```python
from build123d import *

# Parameters (mm, degrees)
SKETCH1_W           = 322.22857931
SKETCH1_H           = 163.1
BOSS_EXTRUDE1_DEPTH = 6.35
SKETCH2_R           = 10.775
CUT_EXTRUDE1_DEPTH  = 362.210727726


with BuildPart() as part:
    # Sketch1 → Boss-Extrude1 (new body)
    with BuildSketch(Plane.XY):
        with Locations((161.114289655, 81.55)):
            Rectangle(SKETCH1_W, SKETCH1_H)
    extrude(amount=BOSS_EXTRUDE1_DEPTH)

    # Sketch2 → Cut-Extrude1 (cut, through all)
    with BuildSketch(Plane.XY.offset(6.35)):
        with Locations((28.8625, 21.55)):
            Circle(SKETCH2_R)
        with Locations((40.366079306, 45.544994544)):
            Circle(SKETCH2_R)
        with Locations((51.8625, 21.55)):
            Circle(SKETCH2_R)
        with Locations((74.8625, 21.55)):
            Circle(SKETCH2_R)
        with Locations((97.8625, 21.55)):
            Circle(SKETCH2_R)
        with Locations((120.8625, 21.55)):
            Circle(SKETCH2_R)
        with Locations((143.8625, 21.55)):
            Circle(SKETCH2_R)
        with Locations((166.8625, 21.55)):
            Circle(SKETCH2_R)
        with Locations((189.8625, 21.55)):
            Circle(SKETCH2_R)
        with Locations((212.8625, 21.55)):
            Circle(SKETCH2_R)
        with Locations((235.8625, 21.55)):
            Circle(SKETCH2_R)
        with Locations((258.8625, 21.55)):
            Circle(SKETCH2_R)
        with Locations((281.8625, 21.55)):
            Circle(SKETCH2_R)
        with Locations((293.366079306, 45.544994544)):
            Circle(SKETCH2_R)
        with Locations((293.366079306, 93.544994544)):
            Circle(SKETCH2_R)
        with Locations((293.366079306, 141.544994544)):
            Circle(SKETCH2_R)
        with Locations((28.8625, 117.55)):
            Circle(SKETCH2_R)
        with Locations((28.8625, 69.55)):
            Circle(SKETCH2_R)
        with Locations((63.366079306, 45.544994544)):
            Circle(SKETCH2_R)
        with Locations((86.366079306, 45.544994544)):
            Circle(SKETCH2_R)
        with Locations((109.366079306, 45.544994544)):
            Circle(SKETCH2_R)
        with Locations((132.366079306, 45.544994544)):
            Circle(SKETCH2_R)
        with Locations((155.366079306, 45.544994544)):
            Circle(SKETCH2_R)
        with Locations((178.366079306, 45.544994544)):
            Circle(SKETCH2_R)
        with Locations((201.366079306, 45.544994544)):
            Circle(SKETCH2_R)
        with Locations((224.366079306, 45.544994544)):
            Circle(SKETCH2_R)
        with Locations((247.366079306, 45.544994544)):
            Circle(SKETCH2_R)
        with Locations((270.366079306, 45.544994544)):
            Circle(SKETCH2_R)
        with Locations((51.8625, 69.55)):
            Circle(SKETCH2_R)
        with Locations((74.8625, 69.55)):
            Circle(SKETCH2_R)
        with Locations((97.8625, 69.55)):
            Circle(SKETCH2_R)
        with Locations((120.8625, 69.55)):
            Circle(SKETCH2_R)
        with Locations((143.8625, 69.55)):
            Circle(SKETCH2_R)
        with Locations((166.8625, 69.55)):
            Circle(SKETCH2_R)
        with Locations((189.8625, 69.55)):
            Circle(SKETCH2_R)
        with Locations((212.8625, 69.55)):
            Circle(SKETCH2_R)
        with Locations((235.8625, 69.55)):
            Circle(SKETCH2_R)
        with Locations((258.8625, 69.55)):
            Circle(SKETCH2_R)
        with Locations((281.8625, 69.55)):
            Circle(SKETCH2_R)
        with Locations((51.8625, 117.55)):
            Circle(SKETCH2_R)
        with Locations((74.8625, 117.55)):
            Circle(SKETCH2_R)
        with Locations((97.8625, 117.55)):
            Circle(SKETCH2_R)
        with Locations((120.8625, 117.55)):
            Circle(SKETCH2_R)
        with Locations((143.8625, 117.55)):
            Circle(SKETCH2_R)
        with Locations((166.8625, 117.55)):
            Circle(SKETCH2_R)
        with Locations((189.8625, 117.55)):
            Circle(SKETCH2_R)
        with Locations((212.8625, 117.55)):
            Circle(SKETCH2_R)
        with Locations((235.8625, 117.55)):
            Circle(SKETCH2_R)
        with Locations((258.8625, 117.55)):
            Circle(SKETCH2_R)
        with Locations((281.8625, 117.55)):
            Circle(SKETCH2_R)
        with Locations((40.366079306, 93.544994544)):
            Circle(SKETCH2_R)
        with Locations((63.366079306, 93.544994544)):
            Circle(SKETCH2_R)
        with Locations((86.366079306, 93.544994544)):
            Circle(SKETCH2_R)
        with Locations((109.366079306, 93.544994544)):
            Circle(SKETCH2_R)
        with Locations((132.366079306, 93.544994544)):
            Circle(SKETCH2_R)
        with Locations((155.366079306, 93.544994544)):
            Circle(SKETCH2_R)
        with Locations((178.366079306, 93.544994544)):
            Circle(SKETCH2_R)
        with Locations((201.366079306, 93.544994544)):
            Circle(SKETCH2_R)
        with Locations((224.366079306, 93.544994544)):
            Circle(SKETCH2_R)
        with Locations((247.366079306, 93.544994544)):
            Circle(SKETCH2_R)
        with Locations((270.366079306, 93.544994544)):
            Circle(SKETCH2_R)
        with Locations((40.366079306, 141.544994544)):
            Circle(SKETCH2_R)
        with Locations((63.366079306, 141.544994544)):
            Circle(SKETCH2_R)
        with Locations((86.366079306, 141.544994544)):
            Circle(SKETCH2_R)
        with Locations((109.366079306, 141.544994544)):
            Circle(SKETCH2_R)
        with Locations((132.366079306, 141.544994544)):
            Circle(SKETCH2_R)
        with Locations((155.366079306, 141.544994544)):
            Circle(SKETCH2_R)
        with Locations((178.366079306, 141.544994544)):
            Circle(SKETCH2_R)
        with Locations((201.366079306, 141.544994544)):
            Circle(SKETCH2_R)
        with Locations((224.366079306, 141.544994544)):
            Circle(SKETCH2_R)
        with Locations((247.366079306, 141.544994544)):
            Circle(SKETCH2_R)
        with Locations((270.366079306, 141.544994544)):
            Circle(SKETCH2_R)
    extrude(amount=-CUT_EXTRUDE1_DEPTH, mode=Mode.SUBTRACT)


solid = part.part
```
Geometry check sheet. Reference: the model listing, model coordinates, mm. Round coordinates to 2 decimals unless told otherwise and drop trailing zeros. Order: outer loops, then holes, each group sorted by start corner. A loop starts at its lowest first (then second) coordinate and runs counter-clockwise, first axis right, second up. Notation, with made-up numbers: (88.25, 72.5) - (108.25, 72.5) arc R7 cw to (108.25, 77.5) - close; hole circle Ø1 at (-29.75, 2). An arc over 180 degrees is marked (long way). Use a Markdown table: item, result. Add a question column.
(1) Sectioned sample at A-A, the plane x = 299. Enter the section's corners in (y, z).
(2) Depth check by flat-ended pin: pin 1 (1.5 mm diameter, centred on x = 236.5, y = 107.5, fed in from +Z). Enter the tip coordinate at first touch or a pass-through.
(3) Sectioned sample at B-B, the plane y = 69.55. Count the separate pieces of the cut face and the enclosed holes in it, and give its area (3 significant figures).
(4) Material ranges on line 1 along Y through (x, z) = (258.5, 4.5); line 2 along Y through (x, z) = (155.5, 1.5), recorded low to high. Write a range as [from, to].
(5) Sectioned sample at C-C, the plane x = 265. Enter the section's corners in (y, z).
(6) Release check for a two-part mould opening along X. For faces 1 (the flat face through (123, 83, 0)), 2 (the cylindrical face through (135.92, 28.83, 3.22)), 3 (the flat face through (0, 80, 3)) record: pulls with the +X half, pulls with the -X half, needs draft (parallel to the pull), parting line crosses it, or undercut.
Answers below:
| question | item | result |
|---|---|---|
| 1 | outline | (0, 0) - (36.36, 0) - (36.36, 6.35) - (0, 6.35) - close; (54.73, 0) - (84.36, 0) - (84.36, 6.35) - (54.73, 6.35) - close; (102.73, 0) - (132.36, 0) - (132.36, 6.35) - (102.73, 6.35) - close; (150.73, 0) - (163.1, 0) - (163.1, 6.35) - (150.73, 6.35) - close |
| 2 | pin 1 | z = 6.35 |
| 3 | separate pieces | 13 |
| 3 | enclosed holes | 0 |
| 3 | area | 404 mm² |
| 4 | line 1 | [0, 10.78], [32.32, 58.78], [80.32, 106.78], [128.32, 163.1] |
| 4 | line 2 | [0, 34.77], [56.32, 82.77], [104.32, 130.77], [152.32, 163.1] |
| 5 | outline | (0, 0) - (12.69, 0) - (12.69, 6.35) - (0, 6.35) - close; (30.41, 0) - (36.2, 0) - (36.2, 6.35) - (30.41, 6.35) - close; (54.89, 0) - (60.69, 0) - (60.69, 6.35) - (54.89, 6.35) - close; (78.41, 0) - (84.2, 0) - (84.2, 6.35) - (78.41, 6.35) - close; (102.89, 0) - (108.69, 0) - (108.69, 6.35) - (102.89, 6.35) - close; (126.41, 0) - (132.2, 0) - (132.2, 6.35) - (126.41, 6.35) - close; (150.89, 0) - (163.1, 0) - (163.1, 6.35) - (150.89, 6.35) - close |
| 6 | face 1 | needs draft |
| 6 | face 2 | undercut |
| 6 | face 3 | pulls with the -X half |
